Source: CAD feature listing. Evaluate the final solid. Frame: model axes, mm. A direction names the side the tool comes from. Coordinates: 2 decimals unless noted, no trailing zeros. Order: outer loops, then holes, each group sorted by start corner. A loop starts at its lowest first (then second) coordinate and runs counter-clockwise, first axis right, second up.
```python
from build123d import *

# Parameters (mm, degrees)
F0_R     = 10
F1_DEPTH = 5
F2_R     = 8
F3_DEPTH = 2
F4_R     = 8
F5_DEPTH = 2
F6_R     = 0.99999


# Not quite as in the source:
# - a fillet or chamfer is up to 0.001 mm smaller than in the source, because OpenCascade refuses the exact size


with BuildPart() as f1:
    # F0 (on Top) → F1 (new body)
    with BuildSketch(Plane.XY):
        Circle(F0_R)
    extrude(amount=F1_DEPTH)

    # F2 (on face) → F3 (join)
    with BuildSketch(Plane(origin=(0, 0, 0), x_dir=(1, 0, 0), z_dir=(0, 0, -1))):
        Circle(F2_R)
    extrude(amount=F3_DEPTH)

    # F4 (on face) → F5 (cut)
    with BuildSketch(Plane.XY.offset(5)):
        Circle(F4_R)
    extrude(amount=-F5_DEPTH, mode=Mode.SUBTRACT)

    # F6 (radius 1 in the source; OpenCascade refuses exactly that, so slightly less here)
    f6_edges = [f1.edges().sort_by_distance(p)[0] for p in [
        (-8, 0, 0),
        (-10, 0, 0),
        (-10, 0, 5),
        (-8, 0, 5),
    ]]
    fillet(f6_edges, radius=F6_R)


solid = f1.part
```
1. Ray query, line 1 (Y direction, x = 0, z = 3.35); line 2 (Z direction, x = 2, y = 2.5); line 3 (X direction, y = 3, z = 4.25). Return the intervals inside material, ascending.
Findings:
line 1: y = -10 to -8, 8 to 10
line 2: z = -2 to 3
line 3: x = -9.51 to -7.45, 7.45 to 9.51
2. Section query D-D on z = 2. Return loops of the section in (x, y).
Findings:
outline: circle Ø20 at (0, 0)
3. Section query C-C on z = 3.25. Return loops of the section in (x, y).
Findings:
outline: circle Ø20 at (0, 0); hole circle Ø16 at (0, 0)
4. Access query for faces 1 (the face through (-1.73, -7.81, 3.51)), 2 (the face through (-1.73, 7.81, -1.49)). Directions: +Z, -Z, +X, -X, +Y, -Y. A direction counts if a zero-diameter tool reaches every point of the face in a straight line with its end or side. Return the directions, or none.
Findings:
face 1: +Z
face 2: -Z
5. Draft query along X for faces 3 (the face through (0, 0, 3)), 4 (the face through (-2.17, -9.76, 2.48)), 5 (the face through (0, 0, -2)). Return one class per face: released by +X, released by -X, zero draft, split by the parting line, or undercut.
Findings:
face 3: undercut
face 4: split by the parting line
face 5: zero draft
6. Pin query (flat end, axial travel): P1, Ø1.5, axis at x = 4.5, z = 3, coming from the +Y side; P2, Ø1, axis at y = -5, z = 0, coming from the +X side; P3, Ø1, axis at x = 2, z = 2, coming from the +Y side. Return the tip coordinate at first contact, or that it passes through.
Findings:
P1: stops at y = 9.27
P2: stops at x = 8.6
P3: stops at y = 9.89
